Check sheet for the drawn part. Datum: minimum x, y, z corner. Units: mm. Coordinates: 2 decimals unless noted, no trailing zeros. Order: outer loops, then holes, each group sorted by start corner. A loop starts at its lowest first (then second) coordinate and runs counter-clockwise, first axis right, second up. Notation, with made-up numbers: (66.25, 12.5) - (99.25, 12.5) arc R30 ccw to (99.25, 35.5) - close; hole circle Ø3 at (-0.5, -13.75). An arc over 180 degrees is marked (long way). Answer as CSV lines item,"result". Start each with the question number.
1. Material ranges on L1, parallel to X at y = 0.55, z = 23.5 (3 decimals); L2, parallel to Z at x = 45, y = 1.7 (3 decimals); L3, parallel to Z at x = 67, y = 2.25 (1 decimal), recorded low to high. Write a range as [from, to].
2. Section check B-B (y = 1.65). Count the separate pieces of the cut face and the enclosed holes in it, and give its area (3 significant figures).
3. Section check D-D (x = 47.5). Record the cut outline in (y, z) (3 decimals), and give its area (3 significant figures).
4. Go/stop test with flat-tipped pins: pin 1 (1 mm diameter, centred on x = 2.5, y = 1, fed in from -Z); pin 2 (1.5 mm diameter, centred on y = 2, z = 66.5, fed in from -X) (3 decimals); pin 3 (1 mm diameter, centred on x = 1.5, y = 2, fed in from +Z). Record where each tip stops, or that it passes through.
5. Section check A-A (z = 68.58). Record the cut outline in (x, y) (3 decimals).
6. Section check C-C (x = 90.5). Record the cut outline in (y, z) (1 decimal), and give its area (3 significant figures).
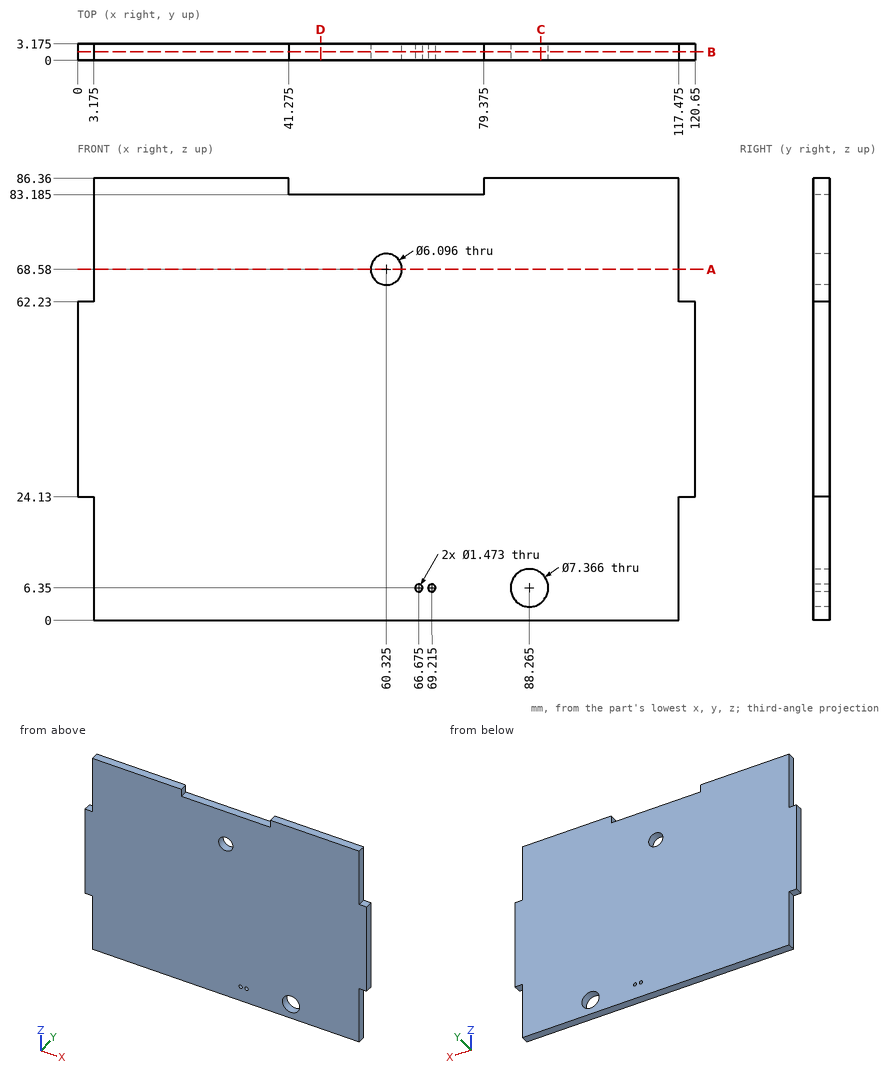
Evaluation:
1,L1,"x = [3.175, 117.475]"
1,L2,"z = [0, 83.185]"
1,L3,"z = [0, 5.7], [7, 83.2]"
2,separate pieces,"1"
2,enclosed holes,"4"
2,area,"9,920 mm²"
3,outline,"(0, 0) - (3.175, 0) - (3.175, 83.185) - (0, 83.185) - close"
3,area,"264 mm²"
4,pin 1,"stops at z = 24.13"
4,pin 2,"stops at x = 3.175"
4,pin 3,"stops at z = 62.23"
5,outline,"(3.175, 0) - (57.277, 0) - (57.277, 3.175) - (3.175, 3.175) - close; (63.373, 0) - (117.475, 0) - (117.475, 3.175) - (63.373, 3.175) - close"
6,outline,"(0, 0) - (3.2, 0) - (3.2, 3.4) - (0, 3.4) - close; (0, 9.3) - (3.2, 9.3) - (3.2, 86.4) - (0, 86.4) - close"
6,area,"256 mm²"
